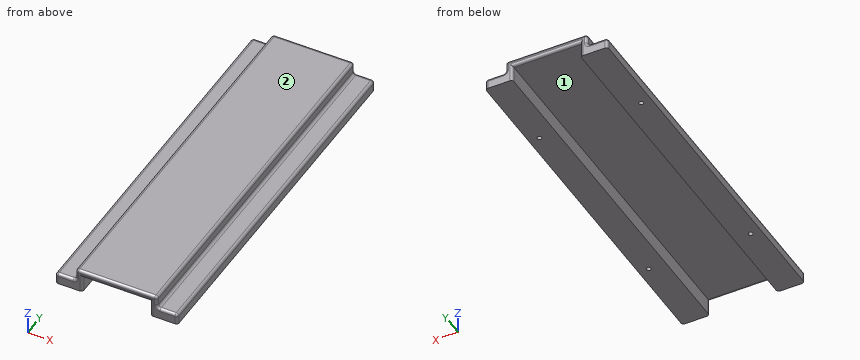
Autodesk Inventor part; units mm, degrees
ref_plane "作業平面1" through (30, 0, 0) normal (1, 0, 0) x (0, 0, -1)
ref_plane "作業平面2" through (0, 135, 0) normal (0, -1, 0) x (1, 0, 0)
ref_plane "YZ Plane" through (0, 0, 0) normal (1, 0, 0) x (0, 1, 0)
sketch "スケッチ1" plane through (0, 0, 0) normal (0, 0, 1) x (1, 0, 0)
  line L0 (0, 0) -> (60, 0)
  line L1 (60, 0) -> (60, 270)
  line L2 (60, 270) -> (0, 270)
  line L3 (0, 270) -> (0, 0)
  dimension "d0" = 270
  dimension "d1" = 60
extrude "押し出し1" add sketch "スケッチ1" along normal blind 17
ref_plane "作業平面1" through (30, 0, 0) normal (1, 0, 0) x (0, 0, -1)
ref_plane "作業平面2" through (0, 135, 0) normal (0, -1, 0) x (1, 0, 0)
sketch "スケッチ2" plane through (0, 0, 0) normal (0, -1, 0) x (1, 0, 0)
  line L0 (30, 24) -> (30, -4)
  line L1 (60, 0) -> (0, 0)
  line L2 (30, 0) -> (5, 0)
  line L3 (5, 0) -> (5, 12)
  line L4 (5, 12) -> (30, 12)
  line L5 (30, 12) -> (30, 0)
  line L6 (0, 17) -> (60, 17)
  line L7 (0, 0) -> (0, 17)
  line L8 (55, 0) -> (55, 12)
  line L9 (55, 12) -> (30, 12)
  point P0 (5, 0)
  dimension "d4" = 5
  dimension "d5" = 5
extrude "押し出し2" cut sketch "スケッチ2" against normal through all contours L9 L8 L1 L0 | L0 L1 L3 L4
sketch "スケッチ3" plane through (0, 0, 17) normal (0, -1, 0) x (1, 0, 0)
  line L0 (5, -17) -> (0, -17)
  line L1 (0, -17) -> (-15, -17)
  line L2 (-15, -17) -> (-15, -9)
  line L3 (-15, -9) -> (0, -9)
  line L4 (0, -9) -> (0, -17)
  line L5 (30, 3.4) -> (30, -20.4)
  line L6 (60, -17) -> (75, -17)
  line L7 (75, -17) -> (75, -9)
  line L8 (75, -9) -> (60, -9)
  line L9 (60, -9) -> (60, -17)
  dimension "d8" = 8
  dimension "d9" = 15
extrude "押し出し3" add sketch "スケッチ3" against normal up to surface (270 mm away)
sketch "スケッチ4" plane through (0, 0, 0) normal (0, 0, 1) x (1, 0, 0)
  line L0 (-15, 0) -> (5, 0)
  line L1 (-15, 0) -> (-15, 270)
  line L2 (30, 324) -> (30, -54)
  line L3 (93, 135) -> (-33, 135)
  point P0 (0, 0)
  point P1 (-7.5, 60)
  point P2 (-7.5, 210)
  point P3 (67.5, 60)
  point P4 (67.5, 210)
  dimension "d12" = 60
  dimension "d13" = 7.5
hole "穴1" at (-7.5, 60, 0) at (-7.5, 210, 0) at (67.5, 60, 0) at (67.5, 210, 0) direction (0, 0, 1) diameter 3.3 depth 5 tip angle 118
fillet "フィレット1" radius 2 26 edges at (30, 0, 17) (30, 0, 12) (5, 0, 6) (55, 0, 6) (60, 0, 12.5) (60, 135, 17) (67.5, 0, 8) (75, 0, 4) (75, 135, 8) (0, 0, 12.5) (-7.5, 0, 8) (-15, 135, 8) (-15, 0, 4) (0, 135, 17) (0, 135, 8) (60, 135, 8) (30, 270, 17) (0, 270, 12.5) (60, 270, 12.5) (67.5, 270, 8) (-7.5, 270, 8) (75, 270, 4) (-15, 270, 4) (30, 270, 12) (55, 270, 6) (5, 270, 6)
properties part number "CableCover"
Can you work these out from the model? Positions are in its coordinate system, mm. Face numbers are marked on the shaded views. Give positions to 0.01 mm unless a question says otherwise; leave off trailing zeros. Order: outer loops, then holes, each group sorted by start corner. A loop starts at its lowest first (then second) coordinate and runs counter-clockwise, first axis right, second up. Notation, with made-up numbers: M 10,44.25 L 32,44.25 A13 cw 32,51.25 Z; hole C -4,3.5 d7. An arc over 180 degrees is marked long. Write item = value, one per line. Start each with the question number.
Q1. I need wall thicknesses on probe 1 along Y at (x, z) = (67.5, 2.55); probe 2 along X at (y, z) = (60, 2.9); probe 3 along X at (y, z) = (53, 1.5). Which ranges of each line are inside material? Lowest first, please. Write a range as [from, to].
Q2. Suppose I cut it at A-A (x = 46). Write out the boundary of the cut face in (y, z).
Q3. We'd pull the mould along X, two halves only. Please class the marked faces 1 and 2: pulls with the +X half, pulls with the -X half, needs draft (parallel to the pull), parting line crosses it, or undercut.
Q4. Will these pins go through, and if not, where does the flat tip stop? pin 1 Ø2.5 at (x, y) = (67.5, 210) entering from -Z; pin 2 Ø2 at (x, y) = (-7.5, 60) entering from +Z; pin 3 Ø9 at (x, y) = (-6, 122.5) entering from +Z.
Q5. Suppose I cut it at B-B (y = 32). Write out the boundary of the cut face in (x, z).
Check result:
q1.probe_1 = [0, 58.35], [61.65, 208.35], [211.65, 270]
q1.probe_2 = [-15, -9.15], [-5.85, 5], [55, 65.85], [69.15, 75]
q1.probe_3 = [-15, 5], [55, 75]
q2.outline = M 0,14 A2 ccw 2,12 L 268,12 A2 ccw 270,14 L 270,15 A2 ccw 268,17 L 2,17 A2 ccw 0,15 Z
q3.face_1 = undercut
q3.face_2 = needs draft
q4.pin_1 = 5.24
q4.pin_2 = 8
q4.pin_3 = 8.06
q5.outline = M -15,0 L 5,0 L 5,12 L 55,12 L 55,0 L 75,0 L 75,6 A2 ccw 73,8 L 62,8 A2 cw 60,10 L 60,15 A2 ccw 58,17 L 2,17 A2 ccw 0,15 L 0,10 A2 cw -2,8 L -13,8 A2 ccw -15,6 Z
